Build history of the part. All positions in model axes, mm. A direction names the side the tool comes from. Round coordinates to 2 decimals unless told otherwise and drop trailing zeros. Write each loop counter-clockwise with the first axis right and the second up, starting at its lowest first coordinate (ties: lowest second). Pieces come first, ordered by that corner, then holes. Notation, with made-up numbers: M -13,48.5 L 10,48.5 A37 cw 10,84.5 Z; hole C 36.25,13.25 d2. An arc over 180 degrees is marked long. Write item = value, one per line.
Autodesk Inventor part; units mm, degrees
ref_plane "YZ Plane" through (0, 0, 0) normal (1, 0, 0) x (0, 1, 0)
ref_plane "XZ Plane" through (0, 0, 0) normal (0, 1, 0) x (-1, 0, 0)
ref_plane "XY Plane" through (0, 0, 0) normal (0, 0, 1) x (1, 0, 0)
sketch "Sketch1" plane through (0, 0, 0) normal (0, 0, 1) x (1, 0, 0)
  line L0 (0, 0) -> (10.5, 0)
  line L1 (10.5, 0) -> (10.5, -5)
  line L2 (10.5, -5) -> (0, -5)
  line L3 (0, -5) -> (0, 0)
  dimension "d0" = 10.5
  dimension "d1" = 5
extrude "Extrusion1" add sketch "Sketch1" along normal blind 3.2
sketch "Sketch2" plane through (0, -5, 0) normal (-1, 0, 0) x (0, 0, 1)
  line L0 (0, 0) -> (0, 5)
  line L1 (0, 2.5) -> (1.6, 2.5)
  circle A0 centre (1.6, 2.5) radius 1.3
  circle A1 centre (1.6, 2.5) radius 2
  point P0 (0, 1.3)
  point P1 (0, 3.7)
  dimension "d4" = 1.6
  dimension "d5" = 2.6
  dimension "d6" = 4
extrude "Extrusion2" add sketch "Sketch2" along normal blind 1.5
extrude "Extrusion3" cut sketch "Sketch2" against normal through all contours A0
move faces "Move1" translate (-0.7, 0, 0) faces at (0, -2.7773, 3.2729)
sketch "Sketch3" plane through (0, 0, 0) normal (0, 0, -1) x (-1, 0, 0)
  line L0 (0, 0) -> (0, -5)
  line L1 (0, -5) -> (0, 0)
  line L2 (0, -2.5) -> (-9.1, -2.5)
  line L3 (-9.1, -2.5) -> (-9.1, -5.6)
  line L4 (-9.1, -5.6) -> (-8.6, -5.6)
  line L5 (-9.1, -5.6) -> (-9.6, -5.6)
  line L6 (-9.6, -5.6) -> (-9.6, -5)
  line L7 (0, -5) -> (-10.5, -5)
  line L8 (-8.6, -5.6) -> (-8.6, -5)
  line L9 (-9.6, -5) -> (-8.6, -5)
  line L10 (-9.1, -5) -> (-5.4, -5)
  line L11 (-5.4, -5) -> (-4.9, -5)
  line L12 (-4.9, -5) -> (-4.9, -5.6)
  line L13 (-4.9, -5.6) -> (-5.9, -5.6)
  line L14 (-5.9, -5.6) -> (-5.9, -5)
  line L15 (-5.4, -5) -> (-1.7, -5)
  line L16 (-1.7, -5) -> (-1.2, -5)
  line L17 (-1.2, -5) -> (-1.2, -5.6)
  line L18 (-1.2, -5.6) -> (-2.2, -5.6)
  line L19 (-2.2, -5.6) -> (-2.2, -5)
  line L20 (-9.1, 0.6) -> (-8.6, 0.6)
  line L21 (-9.1, 0.6) -> (-9.6, 0.6)
  line L22 (-9.6, 0.6) -> (-9.6, 0)
  line L23 (-8.6, 0.6) -> (-8.6, 0)
  line L24 (-9.6, 0) -> (-8.6, 0)
  line L25 (-9.1, 0) -> (-5.4, 0)
  line L26 (-5.4, 0) -> (-4.9, 0)
  line L27 (-4.9, 0) -> (-4.9, 0.6)
  line L28 (-4.9, 0.6) -> (-5.9, 0.6)
  line L29 (-5.9, 0.6) -> (-5.9, 0)
  line L30 (-5.4, 0) -> (-1.7, 0)
  line L31 (-1.7, 0) -> (-1.2, 0)
  line L32 (-1.2, 0) -> (-1.2, 0.6)
  line L33 (-1.2, 0.6) -> (-2.2, 0.6)
  line L34 (-2.2, 0.6) -> (-2.2, 0)
  point P0 (0, -3.7)
  dimension "d14" = 9.1
  dimension "d15" = 3.1
  dimension "d16" = 0.5
  dimension "d17" = 0.5
  dimension "d18" = 3.7
  dimension "d19" = 0.5
  dimension "d20" = 1
  dimension "d21" = 3.7
  dimension "d22" = 0.5
  dimension "d23" = 1
extrude "Extrusion4" add sketch "Sketch3" against normal blind 0.1 contours L17 L18 L19 L7 | L7 L8 L4 L3 | L3 L5 L6 L7 | L7 L12 L13 L14 | L20 L23 L24 L22 L21 | L29 L28 L27 L26 L25 | L34 L33 L32 L31 L30
properties part number "PJ-242"
1. Flat gauge pins, fed straight in: pin 1 (3 mm diameter, centred on x = 4.5, y = -4, fed in from -Z); pin 2 (2 mm diameter, centred on x = 1, z = 1.5, fed in from -Y); pin 3 (1 mm diameter, centred on x = 3, z = 2, fed in from +Y). Where does each tip first touch, or does it go through?
Responses:
pin_1 = 0
pin_2 = -5
pin_3 = 0
2. Probe probe 1 along Y at (x, z) = (3.5, 1.6); probe 2 along Z at (x, y) = (1.75, -2.5); probe 3 along Y at (x, z) = (4.75, 2.1). List the from-to ranges inside material, lowest first.
Responses:
probe_1 = -5 to -3.8, -1.2 to 0
probe_2 = 0 to 0.3, 2.9 to 3.2
probe_3 = -5 to -3.7, -1.3 to 0
3. Band-saw the part on B-B (y = 0.25). List the corners of the cut face in (x, z).
Responses:
outline = M 1.2,0 L 2.2,0 L 2.2,0.1 L 1.2,0.1 Z; M 4.9,0 L 5.9,0 L 5.9,0.1 L 4.9,0.1 Z; M 8.6,0 L 9.6,0 L 9.6,0.1 L 8.6,0.1 Z
4. Band-saw the part on D-D (y = -2.5). List the corners of the cut face in (x, z), plus the area to 3 significant figures.
Responses:
outline = M -1.5,-0.4 L 0,-0.4 L 0,0 L 10.5,0 L 10.5,0.3 L -1.5,0.3 Z; M -1.5,2.9 L 10.5,2.9 L 10.5,3.2 L -0.7,3.2 L -0.7,3.6 L -1.5,3.6 Z
area = 8.12 mm²
5. Band-saw the part on A-A (z = 1.6). List the corners of the cut face in (x, y).
Responses:
outline = M -1.5,-4.5 L 0,-4.5 L 0,-5 L 10.5,-5 L 10.5,-3.8 L -1.5,-3.8 Z; M -1.5,-1.2 L 10.5,-1.2 L 10.5,0 L 0,0 L 0,-0.5 L -1.5,-0.5 Z
6. Tool access for faces 1 (the face through (0, -0.2, 1.6)), 2 (the face through (-0.74, -2.588, -0.398)), 3 (the face through (5, -2, 0)): list every direction of +Z, -Z, +X, -X, +Y, -Y with a clear straight run to the whole face (end or side of a thin tool).
Responses:
face_1 = -X, +Y
face_2 = -X
face_3 = -Z, +X, +Y, -Y
7. Band-saw the part on C-C (x = 1.75). List the corners of the cut face in (y, z).
Responses:
outline = M -5.6,0 L 0.6,0 L 0.6,0.1 L 0,0.1 L 0,3.2 L -5,3.2 L -5,0.1 L -5.6,0.1 Z; hole C -2.5,1.6 d2.6
